Model file for the job. Use its own axes, mm. A direction names the side the tool comes from. Coordinates: 2 decimals unless noted, no trailing zeros. Order: outer loops, then holes, each group sorted by start corner. A loop starts at its lowest first (then second) coordinate and runs counter-clockwise, first axis right, second up.
from build123d import *

# Parameters (mm, degrees)
SKETCH_1_W          = 40
SKETCH_1_H          = 50
SKETCH_1_R          = 1.6
SKETCH_1_R_2        = 3.25
EXTRUDE_1_DEPTH     = 5
SKETCH_2_R          = 13
CUT_EXTRUDE_1_DEPTH = 2.5
SKETCH_3_W          = 40
SKETCH_3_H          = 5
EXTRUDE_2_DEPTH     = 30
SKETCH_4_W          = 25
SKETCH_4_H          = 50
EXTRUDE_3_DEPTH     = 5
FILLET_1_R          = 10


with BuildPart() as part:
    # ｽｹｯﾁ1 → ﾎﾞｽ - 押し出し1 (new body)
    with BuildSketch(Plane.XY):
        Rectangle(SKETCH_1_W, SKETCH_1_H)
        with Locations((0, 8.5)):
            Circle(SKETCH_1_R, mode=Mode.SUBTRACT)
        with Locations((8.5, 0)):
            Circle(SKETCH_1_R, mode=Mode.SUBTRACT)
        with Locations((0, -8.5)):
            Circle(SKETCH_1_R, mode=Mode.SUBTRACT)
        with Locations((-8.5, 0)):
            Circle(SKETCH_1_R, mode=Mode.SUBTRACT)
        Circle(SKETCH_1_R_2, mode=Mode.SUBTRACT)
    extrude(amount=EXTRUDE_1_DEPTH)

    # ｽｹｯﾁ2 → ｶｯﾄ - 押し出し1 (cut)
    with BuildSketch(Plane.XY.offset(5)):
        Circle(SKETCH_2_R)
    extrude(amount=-CUT_EXTRUDE_1_DEPTH, mode=Mode.SUBTRACT)

    # ｽｹｯﾁ3 → ﾎﾞｽ - 押し出し2 (add)
    with BuildSketch(Plane(origin=(0, 0, 0), x_dir=(-1, 0, 0), z_dir=(0, 0, -1))):
        with Locations((0, 27.5)):
            Rectangle(SKETCH_3_W, SKETCH_3_H)
        with Locations((0, -27.5)):
            Rectangle(SKETCH_3_W, SKETCH_3_H)
    extrude(amount=-EXTRUDE_2_DEPTH)

    # ｽｹｯﾁ4 → ﾎﾞｽ - 押し出し3 (add)
    with BuildSketch(Plane(origin=(20, 0, 0), x_dir=(0, 0, -1), z_dir=(1, 0, 0))):
        with Locations((-17.5, 0)):
            Rectangle(SKETCH_4_W, SKETCH_4_H)
    extrude_3 = extrude(amount=-EXTRUDE_3_DEPTH)

    # ﾐﾗｰ1: ﾎﾞｽ - 押し出し3 across plane
    add(extrude_3.mirror(Plane(origin=(0, 0, 0), x_dir=(0, 0, 1), z_dir=(1, 0, 0))))

    # ﾌｨﾚｯﾄ1
    fillet_1_edges = [part.edges().sort_by_distance(p)[0] for p in [
        (15, -25, 17.5),
        (15, 25, 17.5),
        (-15, 25, 17.5),
        (-15, -25, 17.5),
    ]]
    fillet(fillet_1_edges, radius=FILLET_1_R)


solid = part.part
Q1. Cut at B-B, the plane y = 0. List the corners of the cut face in (x, z), plus the area to 3 significant figures.
Established:
outline: (-20, 0) - (-10.1, 0) - (-10.1, 2.5) - (-13, 2.5) - (-13, 5) - (-15, 5) - (-15, 30) - (-20, 30) - close; (-6.9, 0) - (-3.25, 0) - (-3.25, 2.5) - (-6.9, 2.5) - close; (3.25, 0) - (6.9, 0) - (6.9, 2.5) - (3.25, 2.5) - close; (10.1, 0) - (20, 0) - (20, 30) - (15, 30) - (15, 5) - (13, 5) - (13, 2.5) - (10.1, 2.5) - close
area: 353 mm2
Q2. Cut at D-D, the plane x = 8.5. List the corners of the cut face in (y, z).
Established:
outline: (-30, 0) - (-1.6, 0) - (-1.6, 2.5) - (-9.84, 2.5) - (-9.84, 5) - (-24.37, 5) - (-24.37, 30) - (-30, 30) - close; (1.6, 0) - (30, 0) - (30, 30) - (24.37, 30) - (24.37, 5) - (9.84, 5) - (9.84, 2.5) - (1.6, 2.5) - close
Q3. Cut at C-C, the plane z = 10.75. List the corners of the cut face in (x, y).
Established:
outline: (-20, -30) - (20, -30) - (20, 30) - (-20, 30) - close; hole (-15, -15) arc R10 ccw to (-5, -25) - (5, -25) arc R10 ccw to (15, -15) - (15, 15) arc R10 ccw to (5, 25) - (-5, 25) arc R10 ccw to (-15, 15) - close
Q4. Mould opens along X. For faces 3 (the face through (0, -30, 15)), 4 (the face through (3, -3, 2.5)), 5 (the face through (20, 0, 15)) say: pulls with the +X half, pulls with the -X half, needs draft (parallel to the pull), parting line crosses it, or undercut.
Established:
face 3: needs draft
face 4: undercut
face 5: pulls with the +X half
Q5. Probe line 1 (X direction, y = 0, z = 0.7); line 2 (Y direction, x = 0, z = 1.85); line 3 (X direction, y = -3, z = 18.5). List the from-to ranges inside material, lowest first.
Established:
line 1: x = -20 to -10.1, -6.9 to -3.25, 3.25 to 6.9, 10.1 to 20
line 2: y = -30 to -10.1, -6.9 to -3.25, 3.25 to 6.9, 10.1 to 30
line 3: x = -20 to -15, 15 to 20
Q6. Drop flat-ended pins along their axis: P1, Ø15, axis at x = -2, y = -4, coming from the +Z side; P2, Ø3, axis at x = 8.5, y = 0, coming from the -Z side; P3, Ø5, axis at x = -1.5, y = 10.5, coming from the +Z side. Give the stop position or say it passes through.
Established:
P1: stops at z = 2.5
P2: passes through
P3: stops at z = 5
Q7. Cut at A-A, the plane x = 0. List the corners of the cut face in (y, z).
Established:
outline: (-30, 0) - (-10.1, 0) - (-10.1, 2.5) - (-13, 2.5) - (-13, 5) - (-25, 5) - (-25, 30) - (-30, 30) - close; (-6.9, 0) - (-3.25, 0) - (-3.25, 2.5) - (-6.9, 2.5) - close; (3.25, 0) - (6.9, 0) - (6.9, 2.5) - (3.25, 2.5) - close; (10.1, 0) - (30, 0) - (30, 30) - (25, 30) - (25, 5) - (13, 5) - (13, 2.5) - (10.1, 2.5) - close
Q8. Which spindle directions (+Z, -Z, +X, -X, +Y, -Y) get a long thin tool onto all of the face, cutting with end or side? Do faces 1 (the face through (-15, 0, 18)), 2 (the face through (6.9, 0.07, 1.23)). Say none if no direction does.
Established:
face 1: +Z
face 2: +Z, -Z
